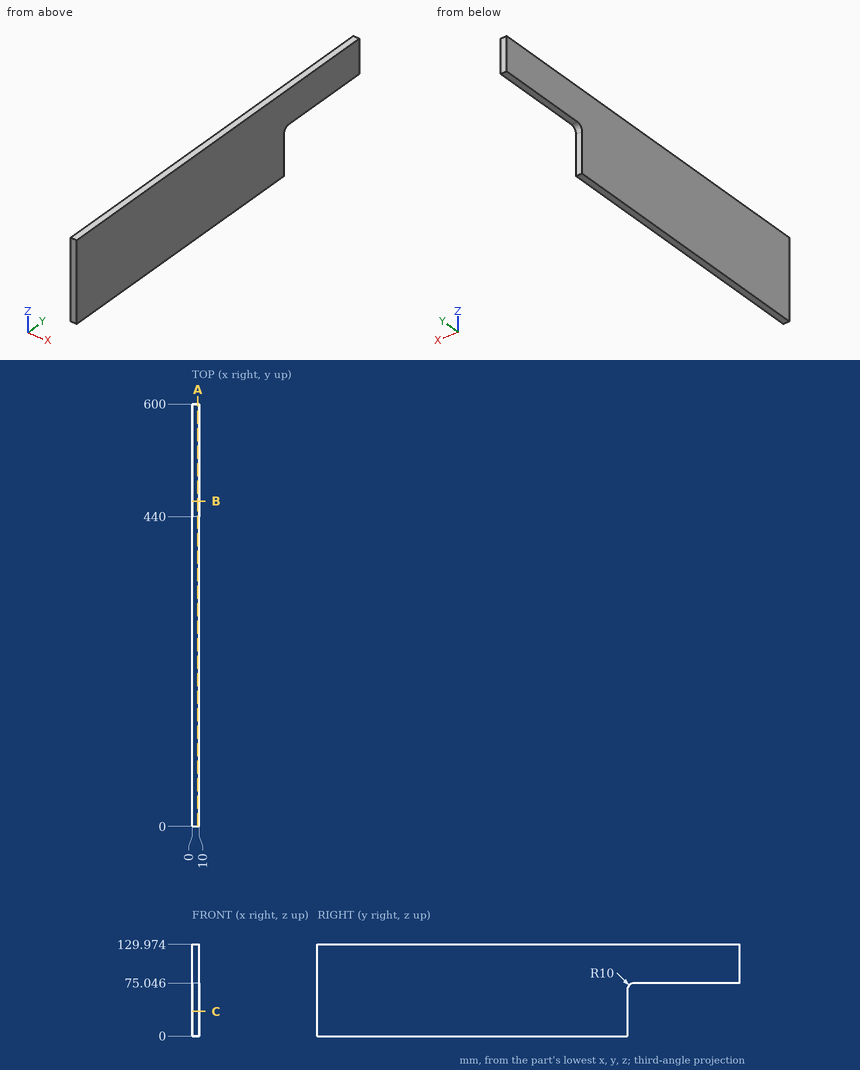
Answer from the drawing. Dimensions are ordinates in mm from the lowest x, y and z of the part. Round coordinates to 2 decimals unless told otherwise and drop trailing zeros. Write each loop counter-clockwise with the first axis right and the second up, starting at its lowest first coordinate (ties: lowest second). Pieces come first, ordered by that corner, then holes. Notation, with made-up numbers: M -10,41 L 32,41 A34 cw 32,71 Z; hole C -25,-1.75 d4. An arc over 180 degrees is marked long. Write each question's results on one line, items separated by ' | '. Start each with the question number.
Item 1: Straight lines are drawn through the part: L1, parallel to Z at x = 1.25, y = 528; L2, parallel to Y at x = 7.75, z = 29. For each, find the intervals that lie inside material, in ascending order. Write a range as [from, to].
Item 2: Flat-ended cylindrical pins translate along their axes: pin 1 Ø2 at (x, z) = (8, 16.5) entering from -Y; pin 2 Ø5 at (x, z) = (3.5, 20.5) entering from +Y. Find the tip coordinate at first contact, or state that the pin passes through.
Item 3: A cutting plane is placed at C-C on z = 35. Write down the section's boundary in (x, y), and give its area (3 significant figures).
Item 4: A cutting plane is placed at B-B on y = 462. Write down the section's boundary in (x, z), and give its area (3 significant figures).
Item 5: A cutting plane is placed at A-A on x = 8. Write down the section's boundary in (y, z).
Check sheet entries:
1) L1: [75.05, 129.97] | L2: [0, 440]
2) pin 1: y = 0 | pin 2: y = 440
3) outline: M 0,0 L 10,0 L 10,440 L 0,440 Z | area: 4,400 mm²
4) outline: M 0,75.05 L 10,75.05 L 10,129.97 L 0,129.97 Z | area: 549 mm²
5) outline: M 0,0 L 440,0 L 440,65.05 A10 cw 450,75.05 L 600,75.05 L 600,129.97 L 0,129.97 Z
